Can you work these out from the model? Positions are in its coordinate system, mm. Face numbers are marked on the shaded views. A direction names the side the tool comes from. Give positions to 0.01 mm unless a question says otherwise; leave off trailing zeros. Loops run counter-clockwise (first coordinate to the right, second up) from the corner with the lowest first, then second, coordinate; pieces in that order, holes last.
from build123d import *

# Parameters (mm, degrees)
F1_DEPTH = 4


with BuildPart() as f1:
    # F0 (on Top) → F1 (new body)
    with BuildSketch(Plane.XY):
        with BuildLine():
            ThreePointArc((1, 1.732051), (1.732051, 1), (2, 0))
            ThreePointArc((2, 0), (-1, -1.732051), (-1, 1.732051))
            Line((-1, 1.732051), (-2.267855, 4.450974))
            Line((-2.267855, 4.450974), (-3.174163, 4.028356))
            Line((-3.174163, 4.028356), (-2.230974, 2.005681))
            ThreePointArc((-2.230974, 2.005681), (0, -3), (2.230974, 2.005681))
            Line((2.230974, 2.005681), (3.174163, 4.028356))
            Line((3.174163, 4.028356), (2.267855, 4.450974))
            Line((2.267855, 4.450974), (1, 1.732051))
        make_face()
    extrude(amount=F1_DEPTH)


solid = f1.part
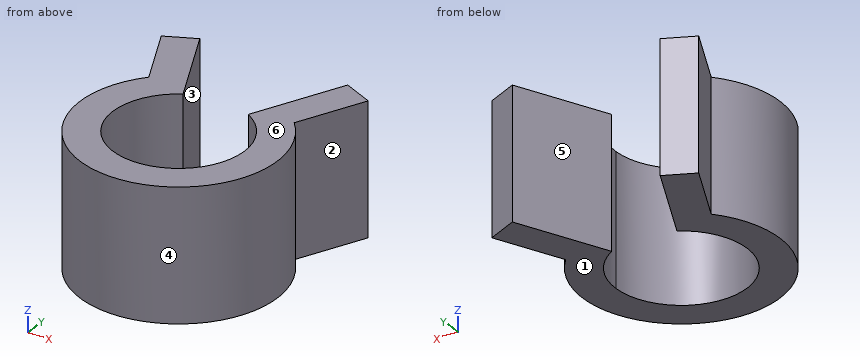
(1) Will these pins go through, and if not, where does the flat tip stop? P1, Ø1, axis at y = 1.5, z = 3, coming from the +X side; P2, Ø1, axis at x = -1, y = -0.5, coming from the -Z side; P3, Ø2, axis at x = 2, z = 1.5, coming from the -Y side.
Returned:
P1: stops at x = 2.83
P2: passes through
P3: stops at y = -2.83
(2) Suppose I cut it at B-B on x = -1.5. List the corners of the cut face in (y, z) for me.
Returned:
outline: (-2.6, 0) - (-1.32, 0) - (-1.32, 4) - (-2.6, 4) - close; (1.32, 0) - (2.8, 0) - (2.8, 4) - (1.32, 4) - close
(3) Which directions (+Z, -Z, +X, -X, +Y, -Y) give clear straight access to the entire face, cutting with the end or side of a thin tool? Please do the marked faces 1, 2 and 3.
Returned:
face 1: -Z, +X, -X, +Y, -Y
face 2: +Z, -Z, +X
face 3: +Z, -Z, +Y
(4) Suppose I cut it at C-C on z = 3.65. List the corners of the cut face in (x, y) for me.
Returned:
outline: (-3.17, 4.03) - (-2.23, 2.01) arc R3 ccw (long way) to (2.23, 2.01) - (3.17, 4.03) - (2.27, 4.45) - (1, 1.73) arc R2 cw (long way) to (-1, 1.73) - (-2.27, 4.45) - close
(5) Suppose I cut it at A-A on y = 3.5. List the corners of the cut face in (x, z) for me, plus the area to 3 significant figures.
Returned:
outline: (-2.93, 0) - (-1.82, 0) - (-1.82, 4) - (-2.93, 4) - close; (1.82, 0) - (2.93, 0) - (2.93, 4) - (1.82, 4) - close
area: 8.83 mm2
(6) Please list where these lines run through material, in increasing order: probe 1 along Y at (x, z) = (0, 1.05); probe 2 along X at (y, z) = (-0.25, 1.35); probe 3 along X at (y, z) = (-0.5, 3.45).
Returned:
probe 1: y = -3 to -2
probe 2: x = -2.99 to -1.98, 1.98 to 2.99
probe 3: x = -2.96 to -1.94, 1.94 to 2.96
(7) Thinking about a two-plate mould opening in X: for the marked faces 4, 5 and 6, which applies, pulls with the +X half, pulls with the -X half, needs draft (parallel to the pull), parting line crosses it, or undercut?
Returned:
face 4: parting line crosses it
face 5: undercut
face 6: needs draft
(8) Suppose I cut it at D-D on x = 0. List the corners of the cut face in (y, z) for me.
Returned:
outline: (-3, 0) - (-2, 0) - (-2, 4) - (-3, 4) - close
